Autodesk Inventor part; units mm, degrees
ref_plane "Work Plane1" through (-9, 0, 0) normal (1, 0, 0) x (0, 1, 0)
ref_plane "XZ Plane" through (0, 0, 0) normal (0, 1, 0) x (-1, 0, 0)
ref_plane "XY Plane" through (0, 0, 0) normal (0, 0, 1) x (1, 0, 0)
sketch "Sketch1" plane through (0, 0, 0) normal (0, 0, 1) x (1, 0, 0)
  circle A0 centre (0, 0) radius 9
  circle A1 centre (-4, 6) radius 1
  circle A2 centre (2, 6) radius 1
  circle A3 centre (2, -6) radius 1
  circle A4 centre (-4, -6) radius 1
  dimension "d0" = 18
  dimension "d2" = 2
  dimension "d3" = 12
  dimension "d4" = 6
  dimension "d6" = 4
  dimension "d7" = 6
  dimension "d8" = 2
  dimension "d15" = 2
extrude "Extrusion1" add sketch "Sketch1" along normal blind 8
sketch "Sketch2" plane through (0, 0, 8) normal (0, 0, -1) x (-1, 0, 0)
  circle A0 centre (0, 0) radius 5
  circle A1 centre (-2, 6) radius 1
  dimension "d11" = 10
extrude "Extrusion2" cut sketch "Sketch2" along normal blind 18 contours A0
ref_plane "Work Plane1" through (-9, 0, 0) normal (1, 0, 0) x (0, 1, 0)
sketch "Sketch3" plane through (-9, 0, 0) normal (1, 0, 0) x (0, 1, 0)
  line L0 (9, 8) -> (-9, 8)
  line L1 (9, 0) -> (-9, 0)
  line L2 (9, 0) -> (9, 8)
  point P0 (0, 0)
  point P1 (0, 4)
  point P2 (9, 4)
  point P3 (0, 0)
hole "Hole1" at (-9, 0, 4) direction (1, 0, 0) diameter 4.134 depth 4.5
properties part number "13"
The listing builds one solid part. Answer for the finished solid, in the listing's coordinates (mm). Coordinates: 2 decimals unless noted, no trailing zeros. Loops run counter-clockwise (first coordinate to the right, second up) from the corner with the lowest first, then second, coordinate; pieces in that order, holes last. Notation, with made-up numbers: (-11.5, 30.25) -> (22.5, 30.25) arc R17 cw to (22.5, 36.25) -> close; hole circle Ø7 at (55.25, -19). An arc over 180 degrees is marked (long way). Write item = value, one per line. Start each with the question number.
1) A cutting plane is placed at A-A (x = 0). Give the vertices of the cut face in (y, z).
2) A cutting plane is placed at D-D (y = 5.75). Give the vertices of the cut face in (x, z), then the cut area to 3 significant figures.
3) Given pin 1 Ø3 at (y, z) = (2, 5) entering from +X; pin 2 Ø3 at (y, z) = (-6.5, 5.5) entering from +X; pin 3 Ø4 at (y, z) = (3.5, 2.5) entering from -X, each flat-ended and moving along its own axis, determine where each tip first touches the part or whether it passes through.
4) The mould has two halves that part along Z. Classify faces 1 (the face through (2, -7, 4)), 2 (the face through (-6.75, 0.79, 5.91)), 3 (the face through (4, -4, 0)): released by +Z, released by -Z, zero draft, split by the parting line, or undercut.
5) A cutting plane is placed at B-B (y = -3.75). Give the vertices of the cut face in (x, z), then the cut area to 3 significant figures.
6) Straight lines are drawn through the part: line 1 (Y direction, x = 0, z = 4.75); line 2 (Y direction, x = 2.25, z = 1.25); line 3 (X direction, y = 0, z = 3.25). For each, find the intervals that lie inside material, in ascending order. Write a range as from..to.
7) A cutting plane is placed at C-C (z = 4.5). Give the vertices of the cut face in (x, y).
Responses:
q1.outline = (-9, 0) -> (-5, 0) -> (-5, 8) -> (-9, 8) -> close; (5, 0) -> (9, 0) -> (9, 8) -> (5, 8) -> close
q2.outline = (-6.92, 0) -> (-4.97, 0) -> (-4.97, 8) -> (-6.92, 8) -> close; (-3.03, 0) -> (1.03, 0) -> (1.03, 8) -> (-3.03, 8) -> close; (2.97, 0) -> (6.92, 0) -> (6.92, 8) -> (2.97, 8) -> close
q2.area = 79.8 mm²
q3.pin_1 = 8.99
q3.pin_2 = 7.48
q3.pin_3 = -8.87
q4.face_1 = zero draft
q4.face_2 = undercut
q4.face_3 = released by -Z
q5.outline = (-8.18, 0) -> (-3.31, 0) -> (-3.31, 8) -> (-8.18, 8) -> close; (3.31, 0) -> (8.18, 0) -> (8.18, 8) -> (3.31, 8) -> close
q5.area = 78.0 mm²
q6.line_1 = -9..-5, 5..9
q6.line_2 = -8.71..-6.97, -5.03..-4.47, 4.47..5.03, 6.97..8.71
q6.line_3 = 5..9
q7.outline = (-8.77, -2.01) arc R9 ccw (long way) to (-8.77, 2.01) -> (-4.58, 2.01) arc R5 cw (long way) to (-4.58, -2.01) -> close; hole circle Ø2 at (-4, -6); hole circle Ø2 at (-4, 6); hole circle Ø2 at (2, -6); hole circle Ø2 at (2, 6)
